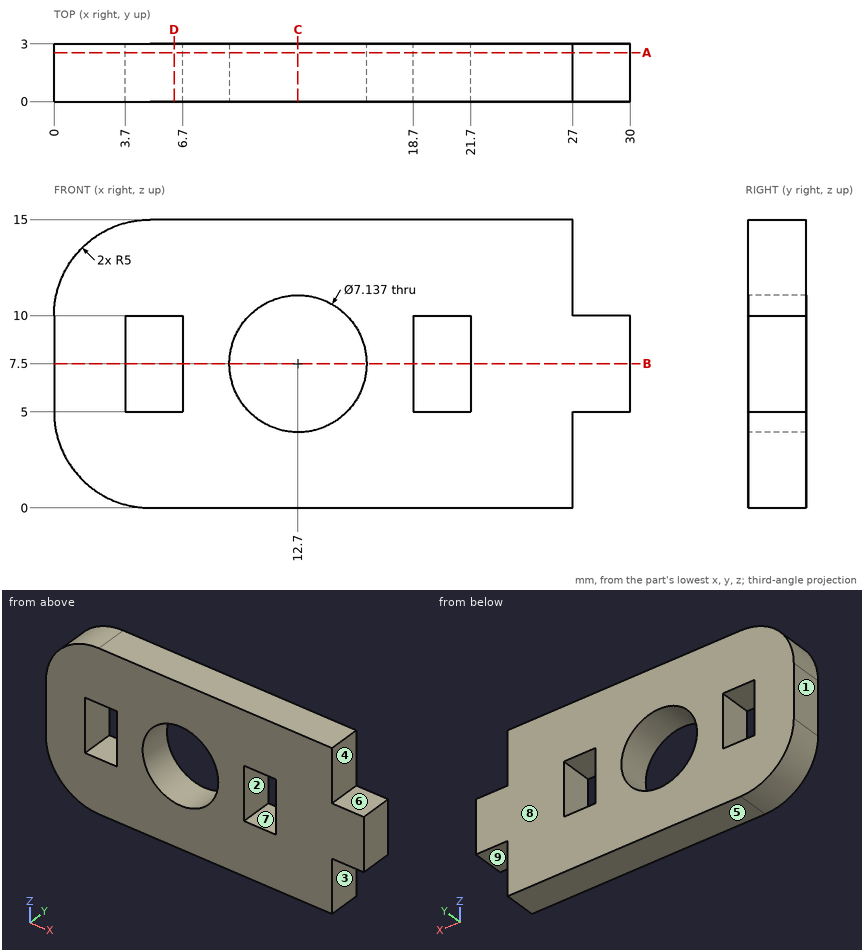
Geometry: see drawing. Coordinates: mm, zero at the bounding-box minimum. A direction names the side the tool comes from. Round coordinates to 2 decimals unless told otherwise and drop trailing zeros. Loops run counter-clockwise (first coordinate to the right, second up) from the corner with the lowest first, then second, coordinate; pieces in that order, holes last. Notation, with made-up numbers: (5.25, -33) - (43.25, -33) arc R22 ccw to (43.25, -14) - close; hole circle Ø2 at (13.5, 53). An arc over 180 degrees is marked (long way). Use CSV: the item, a comma, the result in double quotes.
Q1. Pin query (flat end, axial travel): pin 1 Ø8 at (x, z) = (23, 4) entering from -Y; pin 2 Ø1.5 at (y, z) = (2, 2) entering from +X; pin 3 Ø4.5 at (x, z) = (12.7, 7.5) entering from -Y. Return the tip coordinate at first contact, or that it passes through.
Reported:
pin 1,"y = 0"
pin 2,"x = 27"
pin 3,"through"
Q2. Section query D-D, the plane x = 6.25. Output: boundary loops of the cut face in (y, z).
Reported:
outline,"(0, 0) - (3, 0) - (3, 5) - (0, 5) - close; (0, 10) - (3, 10) - (3, 15) - (0, 15) - close"
Q3. Reachability of the marked faces 1, 2, 3, 4 and 5 from +Z, -Z, +X, -X, +Y, -Y: full face, straight path, thin tool, end or side. Return the list, or none.
Reported:
face 1,"+Z, -Z, -X, +Y, -Y"
face 2,"+Y, -Y"
face 3,"-Z, +X, +Y, -Y"
face 4,"+Z, +X, +Y, -Y"
face 5,"-Z, +X, -X, +Y, -Y"
Q4. Mould query, pull axis Z, two halves, no side actions, for the marked faces 6, 7, 8 and 9. Classes: pulls with the +Z half, pulls with the -Z half, needs draft (parallel to the pull), parting line crosses it, or undercut.
Reported:
face 6,"pulls with the +Z half"
face 7,"undercut"
face 8,"needs draft"
face 9,"pulls with the -Z half"
Q5. Section query B-B, the plane z = 7.5. Output: boundary loops of the cut face in (x, y).
Reported:
outline,"(0, 0) - (3.7, 0) - (3.7, 3) - (0, 3) - close; (6.7, 0) - (9.13, 0) - (9.13, 3) - (6.7, 3) - close; (16.27, 0) - (18.7, 0) - (18.7, 3) - (16.27, 3) - close; (21.7, 0) - (30, 0) - (30, 3) - (21.7, 3) - close"
Q6. Section query A-A, the plane y = 2.55. Output: boundary loops of the cut face in (x, z), then the cut area to 3 significant figures.
Reported:
outline,"(0, 5) arc R5 ccw to (5, 0) - (27, 0) - (27, 5) - (30, 5) - (30, 10) - (27, 10) - (27, 15) - (5, 15) arc R5 ccw to (0, 10) - close; hole (3.7, 5) - (6.7, 5) - (6.7, 10) - (3.7, 10) - close; hole circle Ø7.14 at (12.7, 7.5); hole (18.7, 5) - (21.7, 5) - (21.7, 10) - (18.7, 10) - close"
area,"339 mm^2"
Q7. Section query C-C, the plane x = 12.7. Output: boundary loops of the cut face in (y, z).
Reported:
outline,"(0, 0) - (3, 0) - (3, 3.93) - (0, 3.93) - close; (0, 11.07) - (3, 11.07) - (3, 15) - (0, 15) - close"
Q8. Ray query, line 1 along X through (y, z) = (1.35, 7.5); line 2 along Z through (x, y) = (15.25, 0.7); line 3 along Z through (x, y) = (12.7, 1.3). Return the intervals inside material, ascending.
Reported:
line 1,"0 to 3.7, 6.7 to 9.13, 16.27 to 18.7, 21.7 to 30"
line 2,"0 to 5, 10 to 15"
line 3,"0 to 3.93, 11.07 to 15"
